Geometry: final body of the model. Coordinates: model frame, mm. A direction names the side the tool comes from. Coordinates: 2 decimals unless noted, no trailing zeros. Order: outer loops, then holes, each group sorted by start corner. A loop starts at its lowest first (then second) coordinate and runs counter-clockwise, first axis right, second up. Notation, with made-up numbers: M 54,80 L 87,80 A15 cw 87,97 Z; hole C 11,54 d6. An arc over 180 degrees is marked long. Use CSV: the item, a comma, the result in double quotes. Start each with the question number.
1. Section query C-C on x = -12. Return the cut outline in (y, z) (3 decimals).
2. Section query B-B on x = 0. Return the cut outline in (y, z) (1 decimal), and give its area (3 significant figures).
3. Pull-direction query (X, two-part tool) for faces 1 (the cylindrical face through (-5.658, -1.61, 6.946)), 2 (the flat face through (1.4, -9.525, -1.4)), 3 (the cylindrical face through (-0.69, -6.31, -3.1)); classes: pulls with the +X half, pulls with the -X half, needs draft (parallel to the pull), parting line crosses it, or undercut.
4. Material intervals for line 1 (Z direction, x = 0, y = -1.55); line 2 (Y direction, x = -12.5, z = -3.5) (3 decimals); line 3 (Z direction, x = 10.5, y = -2.5), sorted ascending.
5. Section query A-A on z = 0. Return the cut outline in (x, y) (1 decimal), and give its area (3 significant figures).
6. First-contact query: P1, Ø4, axis at y = -7, z = 2.5, coming from the -X side; P2, Ø1.5, axis at x = 7.5, y = -1.5, coming from the -Z side; P3, Ø3, axis at x = 5.5, z = 7, coming from the -Y side (3 decimals). Flat tips, straight axial feed; report the tip coordinate or a pass-through.
7. Section query D-D on z = 13. Return the cut outline in (x, y) (3 decimals), and give its area (3 significant figures).
8. Set-up query: faces 4 (the cylindrical face through (0.34, 0.78, -1.55)), 5 (the flat face through (0, 1.588, 0)), 6 (the cylindrical face through (-0.34, -7.65, -1.55)). Return all of +Z, -Z, +X, -X, +Y, -Y with unobstructed straight access to the full face (end or side cutting, diameter ignored); none if empty.
from build123d import *

# Parameters (mm, degrees)
F0_R     = 16.66875
F1_DEPTH = 3.175
F2_R     = 3.175
F3_DEPTH = 6.35
F4_R     = 1.5875
F5_DEPTH = 3.81
F6_R     = 2.38125
F7_DEPTH = 25.4
F8_R     = 1.5875
F9_DEPTH = 1.5875


with BuildPart() as f1:
    # F0 (on Front) → F1 (new body)
    with BuildSketch(Plane.XZ):
        Circle(F0_R)
    extrude(amount=F1_DEPTH)

    # F2 (on face) → F3 (join)
    with BuildSketch(Plane.XZ.offset(3.175)):
        Circle(F2_R)
    extrude(amount=F3_DEPTH)

    # F4 (on face) → F5 (cut)
    with BuildSketch(Plane.XZ.offset(9.525)):
        Circle(F4_R)
    extrude(amount=-F5_DEPTH, mode=Mode.SUBTRACT)

    # F6 (on face) → F7 (cut)
    with BuildSketch(Plane.XZ.offset(3.175)):
        with Locations((11.1125, 0)):
            Circle(F6_R)
        with Locations((7.857724, 7.857724)):
            Circle(F6_R)
        with Locations((0, 11.1125)):
            Circle(F6_R)
        with Locations((-7.857724, 7.857724)):
            Circle(F6_R)
        with Locations((-11.1125, 0)):
            Circle(F6_R)
        with Locations((-7.857724, -7.857724)):
            Circle(F6_R)
        with Locations((0, -11.1125)):
            Circle(F6_R)
        with Locations((7.857724, -7.857724)):
            Circle(F6_R)
    extrude(amount=-F7_DEPTH, mode=Mode.SUBTRACT)

    # F8 (on face) → F9 (join)
    with BuildSketch(Plane(origin=(0, 0, 0), x_dir=(-1, 0, 0), z_dir=(0, 1, 0))):
        Circle(F8_R)
    extrude(amount=F9_DEPTH)


solid = f1.part
Results list:
1,outline,"M -3.175,-11.569 L 0,-11.569 L 0,-2.21 L -3.175,-2.21 Z; M -3.175,2.21 L 0,2.21 L 0,11.569 L -3.175,11.569 Z"
2,outline,"M -9.5,-3.2 L -3.2,-3.2 L -3.2,-8.7 L 0,-8.7 L 0,-1.6 L 1.6,-1.6 L 1.6,1.6 L 0,1.6 L 0,8.7 L -3.2,8.7 L -3.2,3.2 L -9.5,3.2 L -9.5,1.6 L -5.7,1.6 L -5.7,-1.6 L -9.5,-1.6 Z; M -3.2,-16.7 L 0,-16.7 L 0,-13.5 L -3.2,-13.5 Z; M -3.2,13.5 L 0,13.5 L 0,16.7 L -3.2,16.7 Z"
2,area,"109 mm²"
3,face 1,"undercut"
3,face 2,"needs draft"
3,face 3,"parting line crosses it"
4,line 1,"z = -16.67 to -13.49, -8.73 to 8.73, 13.49 to 16.67"
4,line 2,"y = -3.175 to 0"
4,line 3,"z = -12.95 to -2.3, 2.3 to 12.95"
5,outline,"M -16.7,-3.2 L -13.5,-3.2 L -13.5,0 L -16.7,0 Z; M -8.7,-3.2 L -3.2,-3.2 L -3.2,-9.5 L -1.6,-9.5 L -1.6,-5.7 L 1.6,-5.7 L 1.6,-9.5 L 3.2,-9.5 L 3.2,-3.2 L 8.7,-3.2 L 8.7,0 L 1.6,0 L 1.6,1.6 L -1.6,1.6 L -1.6,0 L -8.7,0 Z; M 13.5,-3.2 L 16.7,-3.2 L 16.7,0 L 13.5,0 Z"
5,area,"109 mm²"
6,P1,"stops at x = -3.14"
6,P2,"stops at z = -15.24"
6,P3,"stops at y = -3.175"
7,outline,"M -10.433,-3.175 L -1.452,-3.175 L -1.452,0 L -10.433,0 Z; M 1.452,-3.175 L 10.433,-3.175 L 10.433,0 L 1.452,0 Z"
7,area,"57.0 mm²"
8,face 4,"+Y"
8,face 5,"+Z, -Z, +X, -X, +Y"
8,face 6,"-Y"
